Build history of the part. All positions in model axes, mm. A direction names the side the tool comes from. Round coordinates to 2 decimals unless told otherwise and drop trailing zeros. Loops run counter-clockwise (first coordinate to the right, second up) from the corner with the lowest first, then second, coordinate; pieces in that order, holes last. Notation, with made-up numbers: (-8.75, -21) - (48.25, -21) arc R29 cw to (48.25, 17) - close; hole circle Ø3 at (-39, 88.25). An arc over 180 degrees is marked (long way). One line per question, with ' | ' between items. Start each with the question number.
from build123d import *

# Parameters (mm, degrees)
SKETCH1_W           = 63.5
SKETCH1_H           = 57.15
SKETCH1_R           = 12.7
SKETCH1_R_2         = 3.175
BOSS_EXTRUDE2_DEPTH = 4.826
SKETCH2_W           = 53.848
SKETCH2_H           = 57.15
SKETCH2_R           = 6.35
BOSS_EXTRUDE3_DEPTH = 4.826


with BuildPart() as part:
    # Sketch1 → Boss-Extrude2 (new body)
    with BuildSketch(Plane.XY):
        with Locations((0, -3.175)):
            Rectangle(SKETCH1_W, SKETCH1_H)
        Circle(SKETCH1_R, mode=Mode.SUBTRACT)
        with Locations((0, 19.05)):
            Circle(SKETCH1_R_2, mode=Mode.SUBTRACT)
        with Locations((13.470384182, 13.470384182)):
            Circle(SKETCH1_R_2, mode=Mode.SUBTRACT)
        with Locations((19.05, 0)):
            Circle(SKETCH1_R_2, mode=Mode.SUBTRACT)
        with Locations((13.470384182, -13.470384182)):
            Circle(SKETCH1_R_2, mode=Mode.SUBTRACT)
        with Locations((0, -19.05)):
            Circle(SKETCH1_R_2, mode=Mode.SUBTRACT)
        with Locations((-13.470384182, -13.470384182)):
            Circle(SKETCH1_R_2, mode=Mode.SUBTRACT)
        with Locations((-19.05, 0)):
            Circle(SKETCH1_R_2, mode=Mode.SUBTRACT)
        with Locations((-13.470384182, 13.470384182)):
            Circle(SKETCH1_R_2, mode=Mode.SUBTRACT)
    boss_extrude2 = extrude(amount=BOSS_EXTRUDE2_DEPTH)

    # Sketch2 → Boss-Extrude3 (add)
    with BuildSketch(Plane(origin=(31.75, 0, 0), x_dir=(0, 0, -1), z_dir=(1, 0, 0))):
        with Locations((-31.75, -3.175)):
            Rectangle(SKETCH2_W, SKETCH2_H)
        with Locations((-31.75, -3.175)):
            Circle(SKETCH2_R, mode=Mode.SUBTRACT)
    boss_extrude3 = extrude(amount=-BOSS_EXTRUDE3_DEPTH)

    # Mirror1: Boss-Extrude2 across plane
    add(boss_extrude2.mirror(Plane.XY.offset(31.75)))

    # Mirror3: Boss-Extrude3 across plane
    add(boss_extrude3.mirror(Plane.ZY))


solid = part.part
1) Saw through at A-A on z = 31.75. Write the cut outline in (x, y) (3 decimals).
2) Tool access for faces 1 (the flat face through (-26.924, 4, 32)), 2 (the cylindrical face through (15.88, 0.14, 2.38)): list every direction of +Z, -Z, +X, -X, +Y, -Y with a clear straight run to the whole face (end or side of a thin tool).
3) Wall check: line 1 (Y direction, x = 0, z = 59) (3 decimals); line 2 (X direction, y = -3, z = 11.5); line 3 (Y direction, x = -13.5, z = 59). Give the ranges that are in metal, low to high. Write a range as [from, to].
4) Saw through at D-D on z = 22.5. Write the cut outline in (x, y).
5) Two-plate mould, pull along X, no slides. Class faces 3 (the cylindrical face through (16.5, 14.42, 61.12)), 4 (the flat face through (-31.75, 4, 32)), 5 (the flat face through (0, -15, 0)): +X half, -X half, draft (parallel to the pull), parting line (faces both ways), or undercut.
6) Saw through at B-B on y = 19.05. Write the cut outline in (x, z) (3 decimals), and give its area (3 significant figures).
7) Saw through at C-C on x = 0. State how many separate pieces and enclosed holes the cut face has, and give its area (3 significant figures).
Answer key:
1) outline: (-31.75, -31.75) - (-26.924, -31.75) - (-26.924, -9.525) - (-31.75, -9.525) - close; (-31.75, 3.175) - (-26.924, 3.175) - (-26.924, 25.4) - (-31.75, 25.4) - close; (26.924, -31.75) - (31.75, -31.75) - (31.75, -9.525) - (26.924, -9.525) - close; (26.924, 3.175) - (31.75, 3.175) - (31.75, 25.4) - (26.924, 25.4) - close
2) face 1: +Y, -Y | face 2: +Z, -Z
3) line 1: [-31.75, -22.225], [-15.875, -12.7], [12.7, 15.875], [22.225, 25.4] | line 2: [-31.75, -26.92], [26.92, 31.75] | line 3: [-31.75, -16.65], [-10.3, 10.3], [16.65, 25.4]
4) outline: (-31.75, -31.75) - (-26.92, -31.75) - (-26.92, 25.4) - (-31.75, 25.4) - close; (26.92, -31.75) - (31.75, -31.75) - (31.75, 25.4) - (26.92, 25.4) - close
5) face 3: undercut | face 4: -X half | face 5: draft
6) outline: (-31.75, 0) - (-3.175, 0) - (-3.175, 4.826) - (-26.924, 4.826) - (-26.924, 58.674) - (-3.175, 58.674) - (-3.175, 63.5) - (-31.75, 63.5) - close; (3.175, 0) - (31.75, 0) - (31.75, 63.5) - (3.175, 63.5) - (3.175, 58.674) - (26.924, 58.674) - (26.924, 4.826) - (3.175, 4.826) - close | area: 1,070 mm²
7) separate pieces: 8 | enclosed holes: 0 | area: 184 mm²
